Could you check a few things on this model? Use its own coordinates, in mm. Face numbers are marked on the shaded views. A direction names the side the tool comes from. Coordinates: 2 decimals unless noted, no trailing zeros. Order: outer loops, then holes, each group sorted by start corner. A loop starts at its lowest first (then second) coordinate and runs counter-clockwise, first axis right, second up. Notation, with made-up numbers: (2.25, 67) - (59.25, 67) arc R28 ccw to (59.25, 89) - close; hole circle Ø6 at (-39.5, -21.75). An arc over 180 degrees is marked (long way). Answer as a JSON object with one key per item and string values. Group by question number.
(1) Please list where these lines run through material, in increasing order: probe 1 along Y at (x, z) = (31, 2.5); probe 2 along X at (y, z) = (4, 8.5); probe 3 along Y at (x, z) = (3.5, 21).
(2) Imagine slicing it at D-D, the plane y = 5.25. Write out the boundary of the cut face in (x, z).
(3) Imagine slicing it at A-A, the plane z = 9.25. Write out the boundary of the cut face in (x, y), and give its area (3 significant figures).
(4) Will these pins go through, and if not, where does the flat tip stop? P1, Ø6, axis at y = 7, z = 18.5, coming from the +X side; P2, Ø4, axis at x = 22, z = 5, coming from the -Y side; P3, Ø7, axis at x = 5, z = 22, coming from the -Y side.
(5) Imagine slicing it at C-C, the plane y = 18. Write out the boundary of the cut face in (x, z).
(6) Imagine slicing it at B-B, the plane x = 8. Write out the boundary of the cut face in (y, z), and give its area (3 significant figures).
(7) Which directions (+Z, -Z, +X, -X, +Y, -Y) give clear straight access to the entire face, cutting with the end or side of a thin tool? Please do the marked faces 1, 2 and 3.
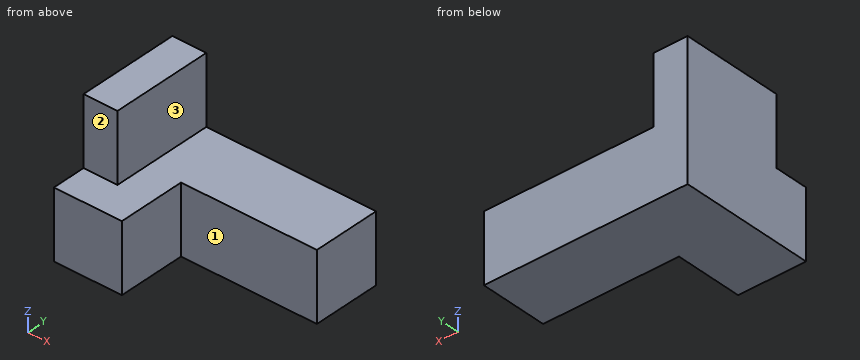
from build123d import *

# Parameters (mm, degrees)
F1_DEPTH = 12.7
F2_W     = 19.05
F2_H     = 12.7
F3_DEPTH = 6.35


with BuildPart() as f1:
    # F0 (on Top) → F1 (new body)
    with BuildSketch(Plane.XY):
        Polygon((38.1, 25.4), (0, 25.4), (0, 0), (12.7, 0), (12.7, 12.7), (38.1, 12.7), align=None)
    extrude(amount=F1_DEPTH)

    # F2 (on face) → F3 (join)
    with BuildSketch(Plane(origin=(0, 0, 0), x_dir=(0, -1, 0), z_dir=(-1, 0, 0))):
        with Locations((-15.875, 19.05)):
            Rectangle(F2_W, F2_H)
    extrude(amount=-F3_DEPTH)


solid = f1.part
Result set:
{
 "1": {"probe 1": "y = 12.7 to 25.4", "probe 2": "x = 0 to 12.7", "probe 3": "y = 6.35 to 25.4"},
 "2": {"outline": "(0, 0) - (12.7, 0) - (12.7, 12.7) - (0, 12.7) - close"},
 "3": {"outline": "(0, 0) - (12.7, 0) - (12.7, 12.7) - (38.1, 12.7) - (38.1, 25.4) - (0, 25.4) - close", "area": "645 mm^2"},
 "4": {"P1": "stops at x = 6.35", "P2": "stops at y = 12.7", "P3": "stops at y = 6.35"},
 "5": {"outline": "(0, 0) - (38.1, 0) - (38.1, 12.7) - (6.35, 12.7) - (6.35, 25.4) - (0, 25.4) - close"},
 "6": {"outline": "(0, 0) - (25.4, 0) - (25.4, 12.7) - (0, 12.7) - close", "area": "323 mm^2"},
 "7": {"face 1": "+Z, -Z, +X, -Y", "face 2": "+Z, +X, -X, -Y", "face 3": "+Z, +X, +Y, -Y"}
}
